```python
from build123d import *

# Parameters (mm, degrees)
SKETCH1_R           = 15
SKETCH1_R_2         = 5.5
BOSS_EXTRUDE1_DEPTH = 8
SKETCH2_R           = 15
SKETCH2_R_2         = 6.5
BOSS_EXTRUDE2_DEPTH = 6
CHAMFER1_SIZE       = 3


with BuildPart() as part:
    # Sketch1 → Boss-Extrude1 (new body)
    with BuildSketch(Plane.XY):
        Circle(SKETCH1_R)
        Circle(SKETCH1_R_2, mode=Mode.SUBTRACT)
    extrude(amount=BOSS_EXTRUDE1_DEPTH)

    # Sketch2 → Boss-Extrude2 (add)
    with BuildSketch(Plane.XY.offset(8)):
        Circle(SKETCH2_R)
        Circle(SKETCH2_R_2, mode=Mode.SUBTRACT)
    extrude(amount=BOSS_EXTRUDE2_DEPTH)

    # Chamfer1
    chamfer1_edges = [part.edges().sort_by_distance(p)[0] for p in [
        (-15, 0, 14),
        (-15, 0, 0),
    ]]
    chamfer(chamfer1_edges, length=CHAMFER1_SIZE)


solid = part.part
```
For this review, take the finished solid that the model builds, in its own axes (mm). A direction names the side the tool comes from. Coordinates: 2 decimals unless noted, no trailing zeros. Order: outer loops, then holes, each group sorted by start corner. A loop starts at its lowest first (then second) coordinate and runs counter-clockwise, first axis right, second up. Notation, with made-up numbers: (63, -0.5) - (122, -0.5) arc R20 ccw to (122, 38.5) - close; hole circle Ø1 at (1.25, -18). An arc over 180 degrees is marked (long way). Answer as a JSON object with one key per item and string values. Group by question number.
1. We need section C-C on z = 3.75. State the section outline as (x, y) points, then the cut area to 3 significant figures.
2. For faces 1 (the flat face through (5.2, -2.5, 0)), 2 (the flat face through (-5, 3, 8)), list the 3-axis set-ups (+Z, -Z, +X, -X, +Y, -Y) from which the entire face can be reached by the end or side of a thin tool; tool diameter is ignored.
3. Clearance check with flat-ended pins moving along their axes: P1, Ø3, axis at x = 10, z = 10.5, coming from the -Y side; P2, Ø8, axis at x = 10, z = 7, coming from the -Y side; P3, Ø1, axis at x = -4, y = -2.5, coming from the +Z side; P4, Ø6, axis at x = -10, z = 2, coming from the +Y side. State where each tip first meets the part, or that it passes through.
4. We need section A-A on y = 0. State the section outline as (x, z) points, then the cut area to 3 significant figures.
5. For probe 1 along Y at (x, z) = (0, 4.5); probe 2 along Y at (x, z) = (0, 9.85); probe 3 along Z at (x, y) = (2.25, 5.5), list the stretches that pass through material, from the lowest coordinate up.
6. The part is to be moulded in two halves that separate along X. For faces 3 (the conical face through (-2.63, -11.86, 13.85)), 4 (the cylindrical face through (-5.158, -3.955, 10.958)), 5 (the flat face through (5, -5, 14)), say which applies: pulls with the +X half, pulls with the -X half, needs draft (parallel to the pull), parting line crosses it, or undercut.
7. We need section D-D on z = 9.5. State the section outline as (x, y) points.
Final values:
{
 "1": {"outline": "circle Ø30 at (0, 0); hole circle Ø11 at (0, 0)", "area": "612 mm²"},
 "2": {"face 1": "-Z, +X, -X, +Y, -Y", "face 2": "+Z"},
 "3": {"P1": "y = -12.36", "P2": "y = -13.75", "P3": "through", "P4": "y = 13.17"},
 "4": {"outline": "(-15, 3) - (-12, 0) - (-5.5, 0) - (-5.5, 8) - (-6.5, 8) - (-6.5, 14) - (-12, 14) - (-15, 11) - close; (5.5, 0) - (12, 0) - (15, 3) - (15, 11) - (12, 14) - (6.5, 14) - (6.5, 8) - (5.5, 8) - close", "area": "236 mm²"},
 "5": {"probe 1": "-15 to -5.5, 5.5 to 15", "probe 2": "-15 to -6.5, 6.5 to 15", "probe 3": "0 to 8"},
 "6": {"face 3": "parting line crosses it", "face 4": "undercut", "face 5": "needs draft"},
 "7": {"outline": "circle Ø30 at (0, 0); hole circle Ø13 at (0, 0)"}
}
